Could you check a few things on this model? Use its own coordinates, in mm. A direction names the side the tool comes from. Give positions to 0.01 mm unless a question says otherwise; leave off trailing zeros. Write each loop counter-clockwise with the first axis right and the second up, starting at its lowest first coordinate (ties: lowest second). Pieces come first, ordered by that corner, then holes. Notation, with made-up numbers: M 3,87 L 40,87 A29 ccw 40,114 Z; hole C 57.5,68.25 d10. An arc over 180 degrees is marked long. Answer as CSV lines item,"result". Start each with the question number.
from build123d import *

# Parameters (mm, degrees)
SKETCH1_W           = 43
SKETCH1_H           = 20
BOSS_EXTRUDE1_DEPTH = 40
SKETCH2_R           = 7.5
BOSS_EXTRUDE2_DEPTH = 15


with BuildPart() as part:
    # Sketch1 → Boss-Extrude1 (new body)
    with BuildSketch(Plane.XY):
        Rectangle(SKETCH1_W, SKETCH1_H)
    extrude(amount=BOSS_EXTRUDE1_DEPTH)

    # Sketch2 → Boss-Extrude2 (add)
    with BuildSketch(Plane.XY.offset(40)):
        with Locations((-11.122255155, 0)):
            Circle(SKETCH2_R)
    extrude(amount=BOSS_EXTRUDE2_DEPTH)


solid = part.part
1. Imagine slicing it at A-A, the plane y = 0. Please give me the cut outline in (x, z), plus the area to 4 significant figures.
2. Imagine slicing it at C-C, the plane x = -8.5. Please give me the cut outline in (y, z).
3. Will these pins go through, and if not, where does the flat tip stop? P1, Ø10, axis at x = -13.5, z = 47.5, coming from the -Y side; P2, Ø6, axis at x = 10, y = -6.5, coming from the +Z side.
4. Please list where these lines run through material, in increasing order: line 1 (Z direction, x = 18.5, y = -8); line 2 (Y direction, x = -16, z = 45.5).
5. On a 3-axis mill with a long thin cutter (end or side, diameter ignored), from which of +Z, -Z, +X, -X, +Y, -Y can I reach the whole of each face in a straight line? I mean faces 1 (the cylindrical face through (-3.969, 2.253, 47.395)), 2 (the flat face through (-11, 0, 55)). Say none if no direction works.
6. Imagine slicing it at B-B, the plane x = 2.5. Please give me the cut outline in (y, z), plus the area to 3 significant figures.
Solutions:
1,outline,"M -21.5,0 L 21.5,0 L 21.5,40 L -3.62,40 L -3.62,55 L -18.62,55 L -18.62,40 L -21.5,40 Z"
1,area,"1,945 mm²"
2,outline,"M -10,0 L 10,0 L 10,40 L 7.03,40 L 7.03,55 L -7.03,55 L -7.03,40 L -10,40 Z"
3,P1,"y = -7.5"
3,P2,"z = 40"
4,line 1,"0 to 40"
4,line 2,"-5.7 to 5.7"
5,face 1,"+Z"
5,face 2,"+Z, +X, -X, +Y, -Y"
6,outline,"M -10,0 L 10,0 L 10,40 L -10,40 Z"
6,area,"800 mm²"
